Here's how the part is built. I have some questions about the finished solid (model axes, mm). A direction names the side the tool comes from. Give positions to 0.01 mm unless a question says otherwise; leave off trailing zeros. Loops run counter-clockwise (first coordinate to the right, second up) from the corner with the lowest first, then second, coordinate; pieces in that order, holes last. Notation, with made-up numbers: M -2,68.5 L 7,68.5 A30 ccw 7,97.5 Z; hole C 10.25,51 d3. An arc over 180 degrees is marked long. Answer as CSV lines item,"result". Start each with the question number.
Item 1: I want a section at A-A on y = 396. List the corners of the cut face in (x, z) for me, plus the area to 3 significant figures.
Item 2: If I drill on line 1 along X through (y, z) = (211.5, 5.25); line 2 along X through (y, z) = (308, 1.75); line 3 along Y through (x, z) = (50.5, 5.5), over which ranges is the centre line in solid material (lowest first)? Write a range as from..to.
Item 3: Will these pins go through, and if not, where does the flat tip stop? P1, Ø1, axis at x = -177, z = -4.5, coming from the -Y side; P2, Ø10, axis at y = 294.5, z = -4.5, coming from the -X side.
Item 4: I want a section at B-B on x = -104.5. List the corners of the cut face in (y, z) for me.
Item 5: If we mould it in two halves opening along X, with no side actions, what happens to faces 1 (the flat face through (299.259, 371.176, 0.21)), 2 (the flat face through (-302.04, 366.36, 0.21)), 3 (the flat face through (3, 540.097, 0)), 4 (the flat face through (429, 192.187, 7))? For each: released by +X, released by -X, zero draft, split by the parting line, or undercut.
Item 6: For faces 5 (the flat face through (-296.66, 369.68, 0.21)), 6 (the flat face through (429, 195.187, 7)), 7 (the flat face through (-429, 195.187, 7)), which set-ups out of +Z, -Z, +X, -X, +Y, -Y let a thin tool reach every point of the face, with its end or its side?
Item 7: I want a section at C-C on x = -378.5. List the corners of the cut face in (y, z) for me.
from build123d import *

# Parameters (mm, degrees)
EXTRUDE_1_DEPTH       = 15
CUT_EXTRUDE_1_REACH   = 576.925
SHEET_START           = -15
SHEET_METAL_2_DEPTH   = 30
SHEET_METAL_2_2_DEPTH = 30


# Read off the part's stored shape, not the designer's step: Преобразовать-Твердое тело2
with BuildPart() as part:
    # Эскиз1 → Вытянуть-Тонкостенный1 (new, symmetric)
    with BuildSketch(Plane.XY):
        with BuildLine():
            Line((-455.166025404, 195.187225691), (-402.598076211, 195.187225691))
            ThreePointArc((-402.598076211, 195.187225691), (-401.098076211, 195.58914948), (-400, 196.687225691))
            Line((-400, 196.687225691), (-200.433012702, 542.347387205))
            ThreePointArc((-200.433012702, 542.347387205), (-199.883974596, 542.896425311), (-199.133974596, 543.097387205))
            Line((-199.133974596, 543.097387205), (199.133974596, 543.097387205))
            ThreePointArc((199.133974596, 543.097387205), (199.883974596, 542.896425311), (200.433012702, 542.347387205))
            Line((200.433012702, 542.347387205), (400, 196.687225691))
            ThreePointArc((400, 196.687225691), (401.098076211, 195.58914948), (402.598076211, 195.187225691))
            Line((402.598076211, 195.187225691), (455.166025404, 195.187225691))
            Line((455.166025404, 195.187225691), (455.166025404, 192.187225691))
            Line((455.166025404, 192.187225691), (402.598076211, 192.187225691))
            ThreePointArc((402.598076211, 192.187225691), (399.598076211, 192.991073269), (397.401923789, 195.187225691))
            Line((397.401923789, 195.187225691), (198.267949192, 540.097387205))
            Line((198.267949192, 540.097387205), (-198.267949192, 540.097387205))
            Line((-198.267949192, 540.097387205), (-397.401923789, 195.187225691))
            ThreePointArc((-397.401923789, 195.187225691), (-399.598076211, 192.991073269), (-402.598076211, 192.187225691))
            Line((-402.598076211, 192.187225691), (-455.166025404, 192.187225691))
            Line((-455.166025404, 192.187225691), (-455.166025404, 195.187225691))
        make_face()
    extrude(amount=EXTRUDE_1_DEPTH, both=True)

    # Эскиз2 → Вырез-Вытянуть1 (cut, up to next)
    with BuildSketch(Plane.XZ.offset(-192.187225691), mode=Mode.PRIVATE) as cut_extrude_1_sk1:
        with BuildLine():
            Line((-445.16238786, -4), (-415.16238786, -4))
            ThreePointArc((-415.16238786, -4), (-411.16238786, 0), (-415.16238786, 4))
            Line((-415.16238786, 4), (-445.16238786, 4))
            ThreePointArc((-445.16238786, 4), (-449.16238786, 0), (-445.16238786, -4))
        make_face()
    cut_extrude_1_tool1 = extrude(cut_extrude_1_sk1.sketch, amount=-CUT_EXTRUDE_1_REACH, mode=Mode.PRIVATE) & part.part
    # Эскиз2 → Вырез-Вытянуть1 (cut, up to next)
    with BuildSketch(Plane.XZ.offset(-192.187225691), mode=Mode.PRIVATE) as cut_extrude_1_sk2:
        with BuildLine():
            Line((445.16238786, 4), (415.16238786, 4))
            ThreePointArc((415.16238786, 4), (411.16238786, 0), (415.16238786, -4))
            Line((415.16238786, -4), (445.16238786, -4))
            ThreePointArc((445.16238786, -4), (449.16238786, 0), (445.16238786, 4))
        make_face()
    cut_extrude_1_tool2 = extrude(cut_extrude_1_sk2.sketch, amount=-CUT_EXTRUDE_1_REACH, mode=Mode.PRIVATE) & part.part
    add(cut_extrude_1_tool1.solids().sort_by_distance((-430.162388, 192.187226, 0))[0], mode=Mode.SUBTRACT)
    add(cut_extrude_1_tool2.solids().sort_by_distance((430.162388, 192.187226, 0))[0], mode=Mode.SUBTRACT)

    # Sheet Metal 2 outline → Sheet Metal 2 (cut)
    with BuildSketch(Plane.XY.offset(SHEET_START)):
        with BuildLine():
            Line((199.133974596, 543.097387205), (197.401923789, 543.097387205))
            ThreePointArc((197.401923789, 543.097387205), (199.651923789, 542.494501522), (201.299038106, 540.847387205))
            Line((201.299038106, 540.847387205), (200.433012702, 542.347387205))
            ThreePointArc((200.433012702, 542.347387205), (199.883974596, 542.896425311), (199.133974596, 543.097387205))
        make_face()
        with BuildLine():
            ThreePointArc((-201.299038106, 540.847387205), (-199.651923789, 542.494501522), (-197.401923789, 543.097387205))
            Line((-197.401923789, 543.097387205), (-199.133974596, 543.097387205))
            ThreePointArc((-199.133974596, 543.097387205), (-199.883974596, 542.896425311), (-200.433012702, 542.347387205))
            Line((-200.433012702, 542.347387205), (-201.299038106, 540.847387205))
        make_face()
    extrude(amount=SHEET_METAL_2_DEPTH, mode=Mode.SUBTRACT)

    # Sheet Metal 2 2 outline → Sheet Metal 2 2 (add)
    with BuildSketch(Plane.XY.offset(SHEET_START)):
        with BuildLine():
            Line((198.267949192, 540.097387205), (197.401923789, 540.097387205))
            ThreePointArc((197.401923789, 540.097387205), (198.151923789, 539.896425311), (198.700961894, 539.347387205))
            Line((198.700961894, 539.347387205), (198.267949192, 540.097387205))
        make_face()
        with BuildLine():
            ThreePointArc((-198.700961894, 539.347387205), (-198.151923789, 539.896425311), (-197.401923789, 540.097387205))
            Line((-197.401923789, 540.097387205), (-198.267949192, 540.097387205))
            Line((-198.267949192, 540.097387205), (-198.700961894, 539.347387205))
        make_face()
    extrude(amount=SHEET_METAL_2_2_DEPTH)


solid = part.part
Result:
1,outline,"M -284.93,-15 L -281.46,-15 L -281.46,15 L -284.93,15 Z; M 281.46,-15 L 284.93,-15 L 284.93,15 L 281.46,15 Z"
1,area,"208 mm^2"
2,line 1,"-391.45..-387.98, 387.98..391.45"
2,line 2,"-335.73..-332.27, 332.27..335.73"
2,line 3,"540.1..543.1"
3,P1,"y = 540.1"
3,P2,"x = -346.41"
4,outline,"M 540.1,-15 L 543.1,-15 L 543.1,15 L 540.1,15 Z"
5,face 1,"released by +X"
5,face 2,"released by -X"
5,face 3,"undercut"
5,face 4,"zero draft"
6,face 5,"+Z, -Z, -Y"
6,face 6,"+Z, -Z, +X, +Y"
6,face 7,"+Z, -Z, -X, +Y"
7,outline,"M 227.93,-15 L 233.93,-15 L 233.93,15 L 227.93,15 Z"
